Input: part model. Units: mm. Frame: model coordinates. Give positions to 0.01 mm unless a question says otherwise; leave off trailing zeros. Write each loop counter-clockwise with the first axis right and the second up, starting at its lowest first coordinate (ties: lowest second). Pieces come first, ordered by that corner, then holes. Notation, with made-up numbers: (-11, 33.25) -> (1, 33.25) arc R22 ccw to (1, 62.25) -> close; hole circle Ø4 at (-18.75, 69). An arc over 180 degrees is marked (long way). Answer as a JSON object with one key per item and string values. Group by question number.
Autodesk Fusion 360 part; units mm, degrees
sketch "Sketch1" plane through (0, 0, 0) normal (1, 0, 0) x (0, 1, 0)
  line L0 (1.725, -1.725) -> (-1.725, -1.725)
  line L1 (-1.725, -1.725) -> (-1.725, 1.725)
  line L2 (-1.725, 1.725) -> (1.725, 1.725)
  line L3 (1.725, 1.725) -> (1.725, -1.725)
  line L4 (1.725, -1.725) -> (-1.725, 1.725) construction
  line L5 (-1.725, -1.725) -> (1.725, 1.725) construction
  dimension "d10" = 3.45
  dimension "d11" = 3.45
extrude "Extrude1" add sketch "Sketch1" along normal blind 4.9
extrude "Extrude2" add 1 faces at (0, -0.575, 0.575) along direction (-1, 0, 0) blind 4.9
fillet "Fillet1" radius 0.4 6 faces at (4.9, -0.575, 0.575) (-4.9, -0.575, 0.575) (1.6333, -0.575, 1.725) (1.6333, -1.725, -0.575) (1.6333, 1.725, 0.575) (1.6333, 0.575, -1.725)
equation "d11 = d10"
1. Section A-A (y = 1.5). Return the cut outline in (x, z) (3 decimals).
2. Contact query for a flat-ended pin moving along its axis: pin 1 Ø2 at (x, z) = (2.5, -1.5) entering from +Y (3 decimals). Output: stop coordinate, or through.
3. Line query: line 1 (Z direction, x = 2, y = -1.45); line 2 (X direction, y = -0.8, z = 1.5); line 3 (Y direction, x = 0.25, z = 1.55). Output: solid intervals per line, ascending.
4. Section B-B (z = 1.45). Return the cut outline in (x, y) (3 decimals), plus the area to 3 significant figures.
Working result:
{
 "1": {"outline": "(-4.86, -1.325) arc R0.36 ccw to (-4.5, -1.685) -> (4.5, -1.685) arc R0.36 ccw to (4.86, -1.325) -> (4.86, 1.325) arc R0.36 ccw to (4.5, 1.685) -> (-4.5, 1.685) arc R0.36 ccw to (-4.86, 1.325) -> close"},
 "2": {"pin 1": "stops at y = 1.725"},
 "3": {"line 1": "z = -1.7 to 1.7", "line 2": "x = -4.86 to 4.86", "line 3": "y = -1.66 to 1.66"},
 "4": {"outline": "(-4.88, -1.325) arc R0.38 ccw to (-4.5, -1.705) -> (4.5, -1.705) arc R0.38 ccw to (4.88, -1.325) -> (4.88, 1.325) arc R0.38 ccw to (4.5, 1.705) -> (-4.5, 1.705) arc R0.38 ccw to (-4.88, 1.325) -> close", "area": "33.2 mm^2"}
}
